Here's how the part is built. I have some questions about the finished solid (model axes, mm). A direction names the side the tool comes from. Round coordinates to 2 decimals unless told otherwise and drop trailing zeros. Order: outer loops, then holes, each group sorted by start corner. A loop starts at its lowest first (then second) coordinate and runs counter-clockwise, first axis right, second up. Notation, with made-up numbers: (87, 79.25) -> (129, 79.25) arc R27 ccw to (129, 114.25) -> close; hole circle Ø11 at (88.25, -37). An arc over 180 degrees is marked (long way). One line per item, written item: value.
```python
from build123d import *

# Parameters (mm, degrees)
SKETCH3_W               = 105.9434
SKETCH3_H               = 211.8868
SKETCH3_W_2             = 18.2245
SKETCH3_H_2             = 105.9434
CUT_EXTRUDE1_DEPTH      = 22.2504
SKETCH5_R               = 6.38175
CUT_EXTRUDE2_DEPTH      = 13.668375
CUT_EXTRUDE2_DEPTH_BACK = 13.668375


with BuildPart() as part:
    # Sketch1 → Revolve1 (revolve)
    with BuildSketch(Plane.XY):
        Polygon((0, 0), (0, 24.80945), (0.762, 25.57145), (5.8166, 25.57145), (6.8707, 24.51735), (7.9248, 24.51735), (7.9248, 26.48585), (29.4386, 26.48585), (30.2006, 25.72385), (30.2006, 0), align=None)
    revolve(axis=Axis((30.2006, 0, 0), (-1, 0, 0)))

    # Sketch2 → Revolve2 (revolve)
    with BuildSketch(Plane.XY):
        with BuildLine():
            Line((30.2006, 0), (30.2006, 17.44345))
            Line((30.2006, 17.44345), (33.4391, 17.44345))
            Line((33.4391, 17.44345), (33.4391, 15.62735))
            ThreePointArc((33.4391, 15.62735), (33.840832339, 14.657482339), (34.8107, 14.25575))
            Line((34.8107, 14.25575), (36.6776, 14.25575))
            ThreePointArc((36.6776, 14.25575), (37.053975321, 14.308400351), (37.401455494, 14.462309321))
            Line((37.401455494, 14.462309321), (37.647467661, 14.61516))
            Line((37.647467661, 14.61516), (38.907307661, 15.875))
            Line((38.907307661, 15.875), (54.31536, 15.875))
            Line((54.31536, 15.875), (55.5752, 14.61516))
            Line((55.5752, 14.61516), (55.5752, 0))
            Line((55.5752, 0), (30.2006, 0))
        make_face()
    revolve(axis=Axis((55.5752, 0, 0), (-1, 0, 0)))

    # Sketch3 → Cut-Extrude1 (cut)
    with BuildSketch(Plane(origin=(55.5752, 0, 0), x_dir=(0, 0, -1), z_dir=(1, 0, 0))):
        Rectangle(SKETCH3_W, SKETCH3_H)
        Rectangle(SKETCH3_W_2, SKETCH3_H_2, mode=Mode.SUBTRACT)
    extrude(amount=-CUT_EXTRUDE1_DEPTH, mode=Mode.SUBTRACT)

    # Sketch4 → Revolve3 (revolve)
    with BuildSketch(Plane.XY):
        with BuildLine():
            Line((6.477090712, 26.401681804), (7.789783697, 25.088988819))
            ThreePointArc((7.789783697, 25.088988819), (7.826981136, 24.999186258), (7.789783697, 24.909383697))
            Line((7.789783697, 24.909383697), (7.39775, 24.51735))
            Line((7.39775, 24.51735), (6.8707, 24.51735))
            Line((6.8707, 24.51735), (6.8707, 24.26335))
            Line((6.8707, 24.26335), (7.9248, 24.26335))
            Line((7.9248, 24.26335), (7.9248, 25.241340712))
            Line((7.9248, 25.241340712), (6.680290712, 26.48585))
            Line((6.680290712, 26.48585), (6.477090712, 26.48585))
            Line((6.477090712, 26.48585), (6.477090712, 26.401681804))
        make_face()
    revolve(axis=Axis((7.9248, 0, 0), (-1, 0, 0)))

    # Sketch5 → Cut-Extrude2 (cut, two sides)
    with BuildSketch(Plane.XY) as cut_extrude2_sk:
        with Locations((44.45, 0)):
            Circle(SKETCH5_R)
    extrude(amount=CUT_EXTRUDE2_DEPTH, mode=Mode.SUBTRACT)
    extrude(cut_extrude2_sk.sketch, amount=-CUT_EXTRUDE2_DEPTH_BACK, mode=Mode.SUBTRACT)

    # Sketch6 → Cut-Revolve1 (revolve, cut)
    with BuildSketch(Plane.XY):
        Polygon((0, 0), (0, 20.5994), (0.762, 19.8374), (3.175, 19.8374), (3.175, 16.59255), (3.937, 15.83055), (12.7, 15.83055), (12.7, 0), align=None)
    revolve(axis=Axis((12.7, 0, 0), (-1, 0, 0)), mode=Mode.SUBTRACT)


solid = part.part
```
Q1. If we mould it in two halves opening along Y, with no side actions, what happens to faces 6 (the face through (45, -7, 9.112)), 7 (the face through (35.757, 14.255, 0.138)), 8 (the face through (1.99, -14.62, -13.41))? For each: pulls with the +Y half, pulls with the -Y half, needs draft (parallel to the pull), parting line crosses it, or undercut.
Answers:
face 6: needs draft
face 7: pulls with the +Y half
face 8: undercut
Q2. I need wall thicknesses on line 1 along Y through (x, z) = (10, 0); line 2 along Y through (x, z) = (2, 0). Which ranges of each line are inside material? Lowest first, please.
Answers:
line 1: -26.49 to -15.83, 15.83 to 26.49
line 2: -25.57 to -19.84, 19.84 to 25.57
Q3. I want a section at A-A on x = 44.45. Write out the boundary of the cut face in (y, z) (3 decimals), then the cut area to 3 significant figures.
Answers:
outline: (-12.999, -9.112) -> (-6.382, -9.112) -> (-6.382, 9.112) -> (-12.999, 9.112) arc R15.875 ccw to start; (6.382, -9.112) -> (12.999, -9.112) arc R15.875 ccw to (12.999, 9.112) -> (6.382, 9.112) -> close
area: 312 mm2
Q4. I want a section at C-C on x = 31.5. Write out the boundary of the cut face in (y, z).
Answers:
outline: circle Ø34.89 at (0, 0)
Q5. I want a section at B-B on x = 5. Write out the boundary of the cut face in (y, z), then the cut area to 3 significant figures.
Answers:
outline: circle Ø51.14 at (0, 0); hole circle Ø31.66 at (0, 0)
area: 1,270 mm2
Q6. Which directions (+Z, -Z, +X, -X, +Y, -Y) give clear straight access to the entire face, cutting with the end or side of a thin tool? Please do faces 1 (the face through (33.439, 16, 0)), 2 (the face through (3.325, 23.622, 9.794)), 3 (the face through (31.84, -3.78, 17.03)), 4 (the face through (46.719, 15.874, 0.136)), 5 (the face through (35.757, -14.255, -0.138)).
Answers:
face 1: +Y
face 2: -X
face 3: +X
face 4: +X, +Y
face 5: -Y
Q7. For P1, Ø6, axis at y = -19.5, z = 6, coming from the +X side; P2, Ø2.5, axis at y = -3.5, z = -15.5, coming from the +X side; P3, Ø9.5, axis at y = -6, z = 0.5, coming from the -X side; P4, Ø7.5, axis at x = 44.45, y = 0, coming from the -Z side (3 decimals), each with a flat end and sliding along its axis, tell me the tip position at first contact or that it passes through.
Answers:
P1: x = 33.44
P2: x = 33.32
P3: x = 12.7
P4: through
